```python
from build123d import *

# Parameters (mm, degrees)
ESTRUSIONE_ESTRUSIONE1_DEPTH = 175
ESTRUSIONE_ESTRUSIONE2_DEPTH = 4
ESTRUSIONE_ESTRUSIONE3_DEPTH = 4
RACCORDO1_R                  = 10
FORO_PER_VITE_M4_1_D         = 4.5
FORO_PER_VITE_M4_1_DEPTH     = 13
FORO_PER_VITE_M4_1_TIP       = 1.351936393
FORO_PER_VITE_M4_2_D         = 4.5
FORO_PER_VITE_M4_2_DEPTH     = 13
FORO_PER_VITE_M4_2_TIP       = 1.351936393


with BuildPart() as part:
    # Schizzo3 → Estrusione-Estrusione1 (new body)
    with BuildSketch(Plane(origin=(0, 0, 0), x_dir=(0, 0, -1), z_dir=(1, 0, 0))):
        Polygon((0, 0), (4, 0), (-6, 10), (-6, 6), align=None)
    extrude(amount=ESTRUSIONE_ESTRUSIONE1_DEPTH)

    # Schizzo4 → Estrusione-Estrusione2 (add)
    with BuildSketch(Plane.XZ):
        Polygon((25, -4), (32.5, -19), (47.5, -19), (55, -4), (120, -4), (127.5, -19), (142.5, -19), (150, -4), (175, -4), (175, 0), (0, 0), (0, -4), align=None)
    extrude(amount=ESTRUSIONE_ESTRUSIONE2_DEPTH)

    # Schizzo5 → Estrusione-Estrusione3 (add)
    with BuildSketch(Plane.XY.offset(6)):
        Polygon((0, 6), (0, 10), (25, 10), (32.5, 25), (47.5, 25), (55, 10), (120, 10), (127.5, 25), (142.5, 25), (150, 10), (175, 10), (175, 6), align=None)
    extrude(amount=ESTRUSIONE_ESTRUSIONE3_DEPTH)

    # Raccordo1
    raccordo1_edges = [part.edges().sort_by_distance(p)[0] for p in [
        (25, -2, -4),
        (32.5, -2, -19),
        (47.5, -2, -19),
        (55, -2, -4),
        (120, -2, -4),
        (127.5, -2, -19),
        (142.5, -2, -19),
        (150, -2, -4),
        (150, 10, 8),
        (142.5, 25, 8),
        (127.5, 25, 8),
        (120, 10, 8),
        (55, 10, 8),
        (47.5, 25, 8),
        (32.5, 25, 8),
        (25, 10, 8),
    ]]
    fillet(raccordo1_edges, radius=RACCORDO1_R)

    # Foro per Vite M4-1
    with Locations(Plane(origin=(0, 0, 0), x_dir=(1, 0, 0), z_dir=(0, 1, 0))):
        with Locations((135, 11), (40, 11)):
            Hole(FORO_PER_VITE_M4_1_D / 2, depth=FORO_PER_VITE_M4_1_DEPTH)
            with Locations((0, 0, -(FORO_PER_VITE_M4_1_DEPTH + FORO_PER_VITE_M4_1_TIP / 2))):  # 118° drill point
                Cone(0, FORO_PER_VITE_M4_1_D / 2, FORO_PER_VITE_M4_1_TIP, mode=Mode.SUBTRACT)

    # Foro per Vite M4-2
    with Locations(Plane(origin=(0, 0, 6), x_dir=(-1, 0, 0), z_dir=(0, 0, -1))):
        with Locations((-40, 17), (-135, 17)):
            Hole(FORO_PER_VITE_M4_2_D / 2, depth=FORO_PER_VITE_M4_2_DEPTH)
            with Locations((0, 0, -(FORO_PER_VITE_M4_2_DEPTH + FORO_PER_VITE_M4_2_TIP / 2))):  # 118° drill point
                Cone(0, FORO_PER_VITE_M4_2_D / 2, FORO_PER_VITE_M4_2_TIP, mode=Mode.SUBTRACT)


solid = part.part
```
The listing builds one solid part. Answer for the finished solid, in the listing's coordinates (mm). A direction names the side the tool comes from. Give positions to 0.01 mm unless a question says otherwise; leave off trailing zeros. Write each loop counter-clockwise with the first axis right and the second up, starting at its lowest first coordinate (ties: lowest second). Pieces come first, ordered by that corner, then holes. Notation, with made-up numbers: (69, 53.25) -> (87, 53.25) arc R25 ccw to (87, 90.25) -> close; hole circle Ø5 at (-14.5, 85.5). An arc over 180 degrees is marked (long way). Write item = value, one per line. Start each with the question number.
1) The part is cut by section B-B, the plane z = 7.5. Determine the outline of the cut face in (x, y).
2) Straight lines are drawn through the part: line 1 along Y through (x, z) = (40, 8.65); line 2 along Z through (x, y) = (40, -2.8); line 3 along X through (y, z) = (-2.3, -11). For each, find the intervals that lie inside material, in ascending order.
3) Each of these flat-tipped pins is pushed along its axis until it touches: pin 1 (2 mm diameter, centred on x = 9.5, y = -1.5, fed in from -Z); pin 2 (6 mm diameter, centred on x = 40, y = 17, fed in from -Z); pin 3 (6 mm diameter, centred on x = 103.5, y = 2.5, fed in from +Z); pin 4 (2.5 mm diameter, centred on x = 40, z = -11, fed in from -Y). Where does it stop, or does it pass through?
4) Determine the mould class of faces 1 (the face through (132.854, -2.028, -11.676)), 2 (the face through (46.511, -2.028, -17.547)), 3 (the face through (89, -2, 0)) for opening direction Z: +Z half, -Z half, draft (parallel to the pull), parting line (faces both ways), or undercut.
5) The part is cut by section A-A, the plane y = 17. Determine the outline of the cut face in (x, z), and give its area (3 significant figures).
6) Which of the six approach directions +Z, -Z, +X, -X, +Y, -Y give full straight-line access (tool end or side, diameter ignored) to faces 4 (the face through (89, 6, 8)), 5 (the face through (40, 14, 6)), 6 (the face through (119.011, 11.453, 8.028)), 7 (the face through (87, -2, -4))?
7) The part is cut by section D-D, the plane z = -6.75. Determine the outline of the cut face in (x, y), and give its area (3 significant figures).
8) The part is cut by section C-C, the plane x = 94. Determine the outline of the cut face in (y, z).
Solutions:
q1.outline = (0, 6) -> (175, 6) -> (175, 10) -> (156.18, 10) arc R10 cw to (147.24, 15.53) -> (145.26, 19.47) arc R10 ccw to (136.32, 25) -> (133.68, 25) arc R10 ccw to (124.74, 19.47) -> (122.76, 15.53) arc R10 cw to (113.82, 10) -> (61.18, 10) arc R10 cw to (52.24, 15.53) -> (50.26, 19.47) arc R10 ccw to (41.32, 25) -> (38.68, 25) arc R10 ccw to (29.74, 19.47) -> (27.76, 15.53) arc R10 cw to (18.82, 10) -> (0, 10) -> close; hole circle Ø4.5 at (40, 17); hole circle Ø4.5 at (135, 17)
q2.line_1 = 6 to 14.75, 19.25 to 25
q2.line_2 = -19 to -13.25, -8.75 to 0
q2.line_3 = 28.5 to 37.75, 42.25 to 51.5, 123.5 to 132.75, 137.25 to 146.5
q3.pin_1 = -4
q3.pin_2 = 6
q3.pin_3 = 5.5
q3.pin_4 = through
q4.face_1 = undercut
q4.face_2 = -Z half
q4.face_3 = +Z half
q5.outline = (28.5, 6) -> (37.75, 6) -> (37.75, 10) -> (28.5, 10) -> close; (42.25, 6) -> (51.5, 6) -> (51.5, 10) -> (42.25, 10) -> close; (123.5, 6) -> (132.75, 6) -> (132.75, 10) -> (123.5, 10) -> close; (137.25, 6) -> (146.5, 6) -> (146.5, 10) -> (137.25, 10) -> close
q5.area = 148 mm²
q6.face_4 = +Z, +X, -X, -Y
q6.face_5 = -Z, +X, -X, +Y
q6.face_6 = +Z, -Z, +Y
q6.face_7 = -Z, +Y, -Y
q7.outline = (25.71, -4) -> (54.29, -4) -> (54.29, 0) -> (25.71, 0) -> close; (120.71, -4) -> (149.29, -4) -> (149.29, 0) -> (120.71, 0) -> close
q7.area = 229 mm²
q8.outline = (-4, -4) -> (0, -4) -> (10, 6) -> (10, 10) -> (6, 10) -> (6, 6) -> (0, 0) -> (-4, 0) -> close
